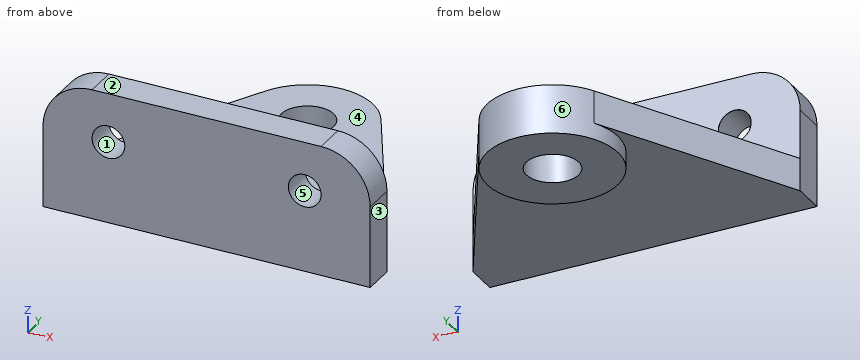
```python
from build123d import *

# Parameters (mm, degrees)
CROQUIS1_W                           = 100
CROQUIS1_H                           = 40
SALIENTE_EXTRUIR1_DEPTH              = 10
CROQUIS2_R                           = 8
SALIENTE_EXTRUIR2_DEPTH              = 10
SALIENTE_EXTRUIR3_START              = -15
CROQUIS3_R                           = 20
CROQUIS3_R_2                         = 8
SALIENTE_EXTRUIR3_DEPTH              = 15
F_10_0_10_DIAMETER_HOLE1_D           = 10
F_10_0_10_DIAMETER_HOLE1_CSINK_D     = 10.05
F_10_0_10_DIAMETER_HOLE1_CSINK_ANGLE = 100
F_10_0_10_DIAMETER_HOLE2_D           = 10
F_10_0_10_DIAMETER_HOLE2_CSINK_D     = 10.05
F_10_0_10_DIAMETER_HOLE2_CSINK_ANGLE = 100
REDONDEO2_R                          = 15


with BuildPart() as part:
    # Croquis1 → Saliente-Extruir1 (new body)
    with BuildSketch(Plane(origin=(0, 0, 0), x_dir=(1, 0, 0), z_dir=(0, 1, 0))):
        with Locations((0, 20)):
            Rectangle(CROQUIS1_W, CROQUIS1_H)
    extrude(amount=SALIENTE_EXTRUIR1_DEPTH)

    # Croquis2 → Saliente-Extruir2 (add)
    with BuildSketch(Plane(origin=(0, 0, -40), x_dir=(-1, 0, 0), z_dir=(0, 0, -1))):
        with BuildLine():
            Line((-17.564659966, 69.564659966), (-50, 10))
            Line((-50, 10), (50, 10))
            Line((50, 10), (17.564659966, 69.564659966))
            ThreePointArc((17.564659966, 69.564659966), (0, 80), (-17.564659966, 69.564659966))
        make_face()
        with Locations((0, 60)):
            Circle(CROQUIS2_R, mode=Mode.SUBTRACT)
    extrude(amount=-SALIENTE_EXTRUIR2_DEPTH)

    # Croquis3 → Saliente-Extruir3 (add)
    with BuildSketch(Plane.XY.offset(-30).offset(SALIENTE_EXTRUIR3_START)):
        with Locations(Location((0, 60, 0), (0, 0, 151.429940189))):
            Circle(CROQUIS3_R)
        with Locations(Location((0, 60, 0), (0, 0, 180))):
            Circle(CROQUIS3_R_2, mode=Mode.SUBTRACT)
    extrude(amount=SALIENTE_EXTRUIR3_DEPTH)

    # Ø10.0 (10) Diameter Hole1 (through all)
    with Locations(Plane(origin=(0, 10, 0), x_dir=(1, 0, 0), z_dir=(0, 1, 0))):
        with Locations((30, 15)):
            CounterSinkHole(F_10_0_10_DIAMETER_HOLE1_D / 2, F_10_0_10_DIAMETER_HOLE1_CSINK_D / 2, counter_sink_angle=F_10_0_10_DIAMETER_HOLE1_CSINK_ANGLE)

    # Ø10.0 (10) Diameter Hole2 (through all)
    with Locations(Plane(origin=(0, 10, 0), x_dir=(1, 0, 0), z_dir=(0, 1, 0))):
        with Locations((-30, 15)):
            CounterSinkHole(F_10_0_10_DIAMETER_HOLE2_D / 2, F_10_0_10_DIAMETER_HOLE2_CSINK_D / 2, counter_sink_angle=F_10_0_10_DIAMETER_HOLE2_CSINK_ANGLE)

    # Redondeo2
    redondeo2_edges = [part.edges().sort_by_distance(p)[0] for p in [
        (50, 5, 0),
        (-50, 5, 0),
    ]]
    fillet(redondeo2_edges, radius=REDONDEO2_R)


solid = part.part
```
Input: part model. Units: mm. Frame: model coordinates. Face numbers are marked on the shaded views. A direction names the side the tool comes from. Round coordinates to 2 decimals unless told otherwise and drop trailing zeros. Loops run counter-clockwise (first coordinate to the right, second up) from the corner with the lowest first, then second, coordinate; pieces in that order, holes last.
1) Set-up query: the marked faces 4, 5 and 6. Return all of +Z, -Z, +X, -X, +Y, -Y with unobstructed straight access to the full face (end or side cutting, diameter ignored); none if empty.
Ans:
face 4: +Z, +X, -X, +Y
face 5: +Y, -Y
face 6: -Z
2) Section query A-A on x = 0. Return the cut outline in (y, z), plus the area to 3 significant figures.
Ans:
outline: (0, -40) - (40, -40) - (40, -45) - (52, -45) - (52, -30) - (10, -30) - (10, 0) - (0, 0) - close; (68, -45) - (80, -45) - (80, -30) - (68, -30) - close
area: 1,060 mm2
3) Material intervals for line 1 (Z direction, x = -30, y = 7.75); line 2 (X direction, y = 60, z = -41.5); line 3 (Y direction, x = 0, z = -35.75), sorted ascending.
Ans:
line 1: z = -40 to -20, -10 to 0
line 2: x = -20 to -8, 8 to 20
line 3: y = 0 to 52, 68 to 80
4) Pin query (flat end, axial travel): pin 1 (11.5 mm diameter, centred on x = 30, z = -15, fed in from +Y); pin 2 (6 mm diameter, centred on y = 62.5, z = -37, fed in from -X); pin 3 (12 mm diameter, centred on y = 42.5, z = -25, fed in from +X). Return the tip coordinate at first contact, or that it passes through.
Ans:
pin 1: stops at y = 10
pin 2: stops at x = -23.05
pin 3: stops at x = 34.11
5) Pull-direction query (X, two-part tool) for the marked faces 1, 2 and 3; classes: released by +X, released by -X, zero draft, split by the parting line, or undercut.
Ans:
face 1: undercut
face 2: zero draft
face 3: released by +X
6) Section query C-C on x = -12.5. Return the cut outline in (y, z), plus the area to 3 significant figures.
Ans:
outline: (0, -40) - (44.39, -40) - (44.39, -45) - (75.61, -45) - (75.61, -30) - (10, -30) - (10, 0) - (0, 0) - close
area: 1,210 mm2
7) Section query B-B on y = 60. Return the cut outline in (x, z), plus the area to 3 significant figures.
Ans:
outline: (-22.77, -40) - (-20, -40) - (-20, -45) - (-8, -45) - (-8, -30) - (-22.77, -30) - close; (8, -45) - (20, -45) - (20, -40) - (22.77, -40) - (22.77, -30) - (8, -30) - close
area: 415 mm2
8) Section query D-D on z = -12. Count the separate pieces of the cut face and the enclosed holes in it, plus the area to 3 significant figures.
Ans:
separate pieces: 3
enclosed holes: 0
area: 834 mm2
